from build123d import *

# Parameters (mm, degrees)
F0_W         = 50
F0_H         = 50
F1_DEPTH     = 55.5
F2_R         = 10
F3_DEPTH     = 25
F4_R         = 24.99999
F5_T1_DEPTH  = 155.50001
F5_T3_DEPTH  = 125.00002
F5_T6_ANGLE  = 90
F5_T8_ANGLE  = 90
F5_T10_ANGLE = 90
F5_T12_ANGLE = 90


# Not quite as in the source:
# - a fillet or chamfer that OpenCascade refuses, or shapes differently, is made with other operations: its cross-section is extruded or revolved along the edge and cut away or added
# - a fillet or chamfer is up to 0.001 mm smaller than in the source, because OpenCascade refuses the exact size


with BuildPart() as f1:
    # F0 (on Top) → F1 (new body)
    with BuildSketch(Plane.XY):
        Rectangle(F0_W, F0_H)
    extrude(amount=F1_DEPTH)

    # F2 (on face) → F3 (cut)
    with BuildSketch(Plane.YZ.offset(25)):
        with Locations((0, 20)):
            Circle(F2_R)
    extrude(amount=-F3_DEPTH, mode=Mode.SUBTRACT)

    # F4 (radius 25 in the source; OpenCascade refuses exactly that, so slightly less here)
    f4_edges = [f1.edges().sort_by_distance(p)[0] for p in [
        (0, -25, 0),
        (0, 25, 0),
    ]]
    fillet(f4_edges, radius=F4_R)

    # F5: fillet of radius 25 on 2 edges, made by hand

    # F5_s2 → F5_t1 (cut)
    with BuildSketch(Plane.XY.offset(-37.50001)):
        with BuildLine():
            ThreePointArc((25, 0), (17.6776695297, -17.6776695297), (0, -25))
            Line((0, -25), (25, -25))
            Line((25, -25), (25, 0))
        make_face()
        with BuildLine():
            ThreePointArc((-25, 0), (-17.6776695297, -17.6776695297), (0, -25))
            Line((0, -25), (-25, -25))
            Line((-25, -25), (-25, 0))
        make_face()
        with BuildLine():
            ThreePointArc((0, 25), (-17.6776695297, 17.6776695297), (-25, 0))
            Line((-25, 0), (-25, 25))
            Line((-25, 25), (0, 25))
        make_face()
        with BuildLine():
            ThreePointArc((0, 25), (17.6776695297, 17.6776695297), (25, 0))
            Line((25, 0), (25, 25))
            Line((25, 25), (0, 25))
        make_face()
    extrude(amount=F5_T1_DEPTH, mode=Mode.SUBTRACT)

    # F5_s4 → F5_t3 (cut)
    with BuildSketch(Plane.XZ.offset(-62.50001)):
        with BuildLine():
            ThreePointArc((-25, 25), (-17.6776695297, 7.3223304703), (0, 0))
            Line((0, 0), (-25, 0))
            Line((-25, 0), (-25, 25))
        make_face()
        with BuildLine():
            ThreePointArc((25, 25), (17.6776695297, 7.3223304703), (0, 0))
            Line((0, 0), (25, 0))
            Line((25, 0), (25, 25))
        make_face()
    extrude(amount=F5_T3_DEPTH, mode=Mode.SUBTRACT)

    # F5_s5 → F5_t6 (revolve, cut)
    with BuildSketch(Plane.XZ.offset(1e-05)):
        with BuildLine():
            ThreePointArc((-25, 24.99999), (-17.6776659941, 7.3223269348), (0, 0))
            Line((0, 0), (-25, 0))
            Line((-25, 0), (-25, 24.99999))
        make_face()
    revolve(axis=Axis((-25, -1e-05, 24.99999), (-1, 0, 0)), revolution_arc=F5_T6_ANGLE, mode=Mode.SUBTRACT)

    # F5_s7 → F5_t8 (revolve, cut)
    with BuildSketch(Plane.XY.offset(24.99999)):
        with BuildLine():
            ThreePointArc((0, 25), (-17.6776659941, 17.6776730652), (-25, 1e-05))
            Line((-25, 1e-05), (-25, 25))
            Line((-25, 25), (0, 25))
        make_face()
    revolve(axis=Axis((-25, 1e-05, 24.99999), (-1, 0, 0)), revolution_arc=F5_T8_ANGLE, mode=Mode.SUBTRACT)

    # F5_s9 → F5_t10 (revolve, cut)
    with BuildSketch(Plane.XZ.offset(1e-05)):
        with BuildLine():
            ThreePointArc((25, 24.99999), (17.6776659941, 7.3223269348), (0, 0))
            Line((0, 0), (25, 0))
            Line((25, 0), (25, 24.99999))
        make_face()
    revolve(axis=Axis((25, -1e-05, 24.99999), (-1, 0, 0)), revolution_arc=F5_T10_ANGLE, mode=Mode.SUBTRACT)

    # F5_s11 → F5_t12 (revolve, cut)
    with BuildSketch(Plane.XY.offset(24.99999)):
        with BuildLine():
            ThreePointArc((25, 1e-05), (17.6776659941, 17.6776730652), (0, 25))
            Line((0, 25), (25, 25))
            Line((25, 25), (25, 1e-05))
        make_face()
    revolve(axis=Axis((25, 1e-05, 24.99999), (-1, 0, 0)), revolution_arc=F5_T12_ANGLE, mode=Mode.SUBTRACT)


solid = f1.part
Could you check a few things on this model? Use its own coordinates, in mm. Round coordinates to 2 decimals unless told otherwise and drop trailing zeros. Order: outer loops, then holes, each group sorted by start corner. A loop starts at its lowest first (then second) coordinate and runs counter-clockwise, first axis right, second up.
(1) Please list where these lines run through material, in increasing order: line 1 along Y through (x, z) = (5.75, 20); line 2 along Z through (x, y) = (1.5, 7); line 3 along Y through (x, z) = (9, 22).
Response values:
line 1: y = -23.81 to -10, 10 to 23.81
line 2: z = 1.05 to 12.86, 27.14 to 55.5
line 3: y = -23.13 to -9.8, 9.8 to 23.13
(2) I'm going to push flat-ended pins straight in: pin 1 (1 mm diameter, centred on x = 11.5, z = 35.5, fed in from -Y); pin 2 (10 mm diameter, centred on y = 14, z = 13.5, fed in from +X); pin 3 (8 mm diameter, centred on x = -6.5, z = 18, fed in from -Y); pin 4 (12 mm diameter, centred on y = 0, z = 20, fed in from -X). Where does each tip first touch, or does it pass through?
Response values:
pin 1: stops at y = -22.45
pin 2: stops at x = 21.28
pin 3: stops at y = -24.38
pin 4: stops at x = -25
(3) Imagine slicing it at B-B (z = 28). Write out the boundary of the cut face in (x, y), plus the area to 3 significant figures.
Response values:
outline: (0, -6) - (0, 6) - (24.27, 6) arc R25 ccw (long way) to (24.27, -6) - close
area: 1,670 mm2
(4) Imagine slicing it at A-A (z = 51.5). Write out the boundary of the cut face in (x, y).
Response values:
outline: circle Ø50 at (0, 0)
(5) If we mould it in two halves opening along Z, with no side actions, what happens to faces 1 (the cylindrical face through (12.675, -1.302, 29.915)), 2 (the flat face through (0, 0, 55.5))? For each: released by +Z, released by -Z, zero draft, split by the parting line, or undercut.
Response values:
face 1: undercut
face 2: released by +Z
